from build123d import *

# Parameters (mm, degrees)
SKETCH1_R            = 19.1
BOSS_EXTRUDE1_DEPTH  = 33.25
SKETCH2_R            = 7.8
SKETCH2_R_2          = 4
BOSS_EXTRUDE2_DEPTH  = 6.75
BOSS_EXTRUDE4_DEPTH  = 7.5
CUT_EXTRUDE1_REACH   = 54.523
FILLET1_R            = 1
FILLET1_OF_MIRROR2_R = 1
CUT_EXTRUDE2_START   = -6.85
SKETCH2_3_R          = 4
CUT_EXTRUDE2_DEPTH   = 13.6
BOSS_EXTRUDE5_DEPTH  = 30
FILLET2_R            = 6
SKETCH6_R            = 2.5
BOSS_EXTRUDE6_DEPTH  = 40


with BuildPart() as part:
    # Sketch1 → Boss-Extrude1 (new body)
    with BuildSketch(Plane.XY):
        Circle(SKETCH1_R)
    extrude(amount=-BOSS_EXTRUDE1_DEPTH)

    # Sketch2 → Boss-Extrude2 (add)
    with BuildSketch(Plane.XY):
        Circle(SKETCH2_R)
        Circle(SKETCH2_R_2, mode=Mode.SUBTRACT)
    extrude(amount=BOSS_EXTRUDE2_DEPTH)

    # Sketch3 → Boss-Extrude4 (add, symmetric)
    with BuildSketch(Plane(origin=(0, 0, 0), x_dir=(1, 0, 0), z_dir=(0, 1, 0))):
        Polygon((26.7, -6.95), (26.7, -7.75), (16.12, -7.75), (16.12, -0.2), (0, -0.2), (0, 0), (16.4, 0), (16.4, -6.95), align=None)
    boss_extrude4 = extrude(amount=BOSS_EXTRUDE4_DEPTH, both=True)

    # Sketch4 → Cut-Extrude1 (cut, up to next)
    with BuildSketch(Plane.XY.offset(7.75), mode=Mode.PRIVATE) as cut_extrude1_sk1:
        with BuildLine():
            ThreePointArc((25.0538758, -4.749032258), (25.5, 0), (25.0538758, 4.749032258))
            ThreePointArc((25.0538758, 4.749032258), (22.424207442, 6.5406361), (20.6326036, 3.910967742))
            ThreePointArc((20.6326036, 3.910967742), (21, 0), (20.6326036, -3.910967742))
            ThreePointArc((20.6326036, -3.910967742), (22.424207442, -6.5406361), (25.0538758, -4.749032258))
        make_face()
    cut_extrude1_tool1 = extrude(cut_extrude1_sk1.sketch, amount=-CUT_EXTRUDE1_REACH, mode=Mode.PRIVATE) & part.part
    # Sketch4 → Cut-Extrude1 (cut, up to next)
    with BuildSketch(Plane.XY.offset(7.75), mode=Mode.PRIVATE) as cut_extrude1_sk2:
        with BuildLine():
            ThreePointArc((26.7, -1.8e-08), (26.461554926, -3.779963633), (25.75, -7.5))
            Line((25.75, -7.5), (26.7, -7.5))
            Line((26.7, -7.5), (26.7, -1.8e-08))
        make_face()
    cut_extrude1_tool2 = extrude(cut_extrude1_sk2.sketch, amount=-CUT_EXTRUDE1_REACH, mode=Mode.PRIVATE) & part.part
    # Sketch4 → Cut-Extrude1 (cut, up to next)
    with BuildSketch(Plane.XY.offset(7.75), mode=Mode.PRIVATE) as cut_extrude1_sk3:
        with BuildLine():
            ThreePointArc((25.75, 7.5), (26.461554929, 3.779963615), (26.7, -1.8e-08))
            Line((26.7, -1.8e-08), (26.7, 7.5))
            Line((26.7, 7.5), (25.75, 7.5))
        make_face()
    cut_extrude1_tool3 = extrude(cut_extrude1_sk3.sketch, amount=-CUT_EXTRUDE1_REACH, mode=Mode.PRIVATE) & part.part
    cut_extrude1_1 = cut_extrude1_tool1.solids().sort_by_distance((23.036032, 0, 7.75))[0]
    add(cut_extrude1_1, mode=Mode.SUBTRACT)
    cut_extrude1_2 = cut_extrude1_tool2.solids().sort_by_distance((26.415788, -5.630973, 7.75))[0]
    add(cut_extrude1_2, mode=Mode.SUBTRACT)
    cut_extrude1_3 = cut_extrude1_tool3.solids().sort_by_distance((26.415788, 5.630973, 7.75))[0]
    add(cut_extrude1_3, mode=Mode.SUBTRACT)
    cut_extrude1 = cut_extrude1_1 + cut_extrude1_2 + cut_extrude1_3  # Cut-Extrude1 as one shape, for the pattern or mirror that repeats it

    # Fillet1
    fillet1_edges = [part.edges().sort_by_distance(p)[0] for p in [
        (25.75, -7.5, 7.35),
        (25.75, 7.5, 7.35),
    ]]
    fillet(fillet1_edges, radius=FILLET1_R)

    # Mirror2: Boss-Extrude4, Cut-Extrude1 across plane
    add(boss_extrude4.mirror(Plane(origin=(0, 0, 0), x_dir=(0, 0, 1), z_dir=(1, 0, 0))))
    add(cut_extrude1.mirror(Plane(origin=(0, 0, 0), x_dir=(0, 0, 1), z_dir=(1, 0, 0))), mode=Mode.SUBTRACT)

    # Fillet1 of Mirror2
    fillet1_of_mirror2_edges = [part.edges().sort_by_distance(p)[0] for p in [
        (-25.75, -7.5, 7.35),
        (-25.75, 7.5, 7.35),
    ]]
    fillet(fillet1_of_mirror2_edges, radius=FILLET1_OF_MIRROR2_R)

    # Sketch2<3> → Cut-Extrude2 (cut)
    with BuildSketch(Plane.XY.offset(CUT_EXTRUDE2_START)):
        Circle(SKETCH2_3_R)
    extrude(amount=CUT_EXTRUDE2_DEPTH, mode=Mode.SUBTRACT)

    # Sketch5 → Boss-Extrude5 (add)
    with BuildSketch(Plane(origin=(0, 0, 0), x_dir=(0, 0, 1), z_dir=(0.17364817766693072, 0.984807753012208, 0))):
        Polygon((-31.25, -3.492969129), (-25.2, -6.985938257), (-19.15, -3.492969129), (-19.15, 3.492969129), (-25.2, 6.985938257), (-31.25, 3.492969129), align=None)
    extrude(amount=BOSS_EXTRUDE5_DEPTH)

    # Fillet2
    fillet2_edges = [part.edges().sort_by_distance(p)[0] for p in [
        (5.20944533, 29.54423259, -31.25),
        (0.049590712, 30.454054176, -28.225),
        (0.049590712, 30.454054176, -22.175),
        (5.20944533, 29.54423259, -19.15),
        (10.369299948, 28.634411005, -22.175),
        (10.369299948, 28.634411005, -28.225),
    ]]
    fillet(fillet2_edges, radius=FILLET2_R)

    # Sketch6 → Boss-Extrude6 (add)
    with BuildSketch(Plane(origin=(0, 0, 0), x_dir=(0, 0, 1), z_dir=(0.17364817766693072, 0.984807753012208, 0))):
        with Locations(Location((-25.2, 0, 0), (0, 0, 90))):
            Circle(SKETCH6_R)
    extrude(amount=BOSS_EXTRUDE6_DEPTH)


solid = part.part
Geometry: final body of the model. Coordinates: model frame, mm. A direction names the side the tool comes from. Round coordinates to 2 decimals unless told otherwise and drop trailing zeros. Loops run counter-clockwise (first coordinate to the right, second up) from the corner with the lowest first, then second, coordinate; pieces in that order, holes last. Notation, with made-up numbers: (78.25, 56) - (86.25, 56) arc R28 ccw to (86.25, 87) - close; hole circle Ø10 at (73, 31.5). An arc over 180 degrees is marked (long way). Write each question's results on one line, items separated by ' | '. Start each with the question number.
1) Line query: probe 1 along Z at (x, y) = (-17.5, 0); probe 2 along Z at (x, y) = (13.5, -8); probe 3 along Y at (x, z) = (0, -3). Output: solid intervals per line, ascending. Write a range as [from, to].
2) Cut plane C-C on y = -11. Return loops of the section in (x, z), then the cut area to 3 significant figures.
3) Cut plane B-B on z = -6. Return loops of the section in (x, y).
4) Access query for faces 4 (the face through (-20, 0, 6.95)), 5 (the face through (20, 0, 6.95)), 6 (the face through (-4, 2, 6.75)). Directions: +Z, -Z, +X, -X, +Y, -Y. A direction counts if a zero-diameter tool reaches every point of the face in a straight line with its end or side. Return the directions, or none.
5) First-contact query: P1, Ø6.5, axis at x = 2, y = -0.5, coming from the +Z side; P2, Ø4, axis at x = -17, z = 4, coming from the +Y side; P3, Ø10, axis at x = 10, y = 27, coming from the +Z side; P4, Ø3, axis at x = -4.5, y = 27.5, coming from the +Z side. Flat tips, straight axial feed; report the tip coordinate or a pass-through.
6) Cut plane A-A on x = -22.5. Return loops of the section in (y, z), then the cut area to 3 significant figures.
7) Mould query, pull axis Z, two halves, no side actions, for faces 1 (the face through (0, 0, -6.85)), 2 (the face through (16.4, 0, 3)), 3 (the face through (8.804, 19.614, -28.183)). Classes: released by +Z, released by -Z, zero draft, split by the parting line, or undercut.
Verdict:
1) probe 1: z = [-33.25, 0], [6.95, 7.75] | probe 2: z = [-33.25, 0] | probe 3: y = [-19.1, -4], [4, 19.1]
2) outline: (-15.61, -33.25) - (15.61, -33.25) - (15.61, 0) - (-15.61, 0) - close | area: 1,040 mm2
3) outline: circle Ø38.2 at (0, 0); hole circle Ø8 at (0, 0)
4) face 4: -X, +Y, -Y | face 5: +X, +Y, -Y | face 6: +Z, +Y, -Y
5) P1: stops at z = 6.75 | P2: stops at y = 7.5 | P3: stops at z = -19.15 | P4: passes through
6) outline: (-7.5, 6.95) - (-6.55, 6.95) - (-6.55, 7.75) - (-7.5, 7.75) - close; (6.55, 6.95) - (7.5, 6.95) - (7.5, 7.75) - (6.55, 7.75) - close | area: 1.51 mm2
7) face 1: released by +Z | face 2: undercut | face 3: released by -Z
